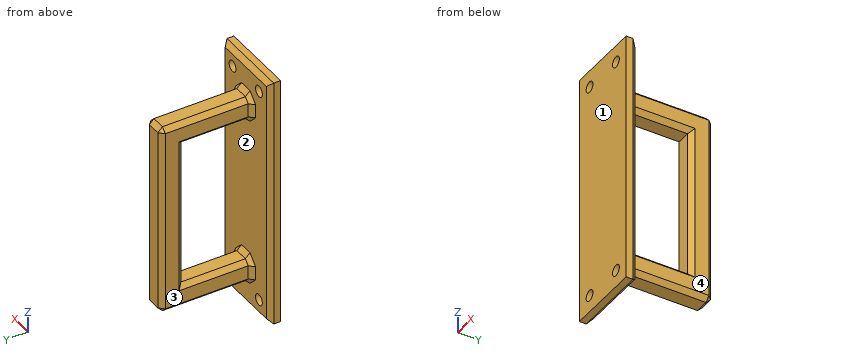
from build123d import *

# Parameters (mm, degrees)
SKETCH1_W           = 41.91
SKETCH1_H           = 139.7
BOSS_EXTRUDE1_DEPTH = 6.35
SKETCH2_R           = 3.048
CUT_EXTRUDE1_DEPTH  = 146.989248234
SKETCH3_W           = 12.7
SKETCH3_H           = 12.7
BOSS_EXTRUDE2_DEPTH = 50.8
BOSS_EXTRUDE3_REACH = 133.265
SKETCH4_W           = 12.7
SKETCH4_H           = 12.7
CHAMFER1_SIZE       = 2.54


with BuildPart() as part:
    # Sketch1 → Boss-Extrude1 (new body)
    with BuildSketch(Plane(origin=(0, 0, 0), x_dir=(1, 0, 0), z_dir=(0, 1, 0))):
        with Locations((-20.955, 69.85)):
            Rectangle(SKETCH1_W, SKETCH1_H)
    extrude(amount=BOSS_EXTRUDE1_DEPTH)

    # Sketch2 → Cut-Extrude1 (cut, through all)
    with BuildSketch(Plane(origin=(0, 6.35, 0), x_dir=(1, 0, 0), z_dir=(0, 1, 0))):
        with Locations(Location((-32.766, 130.302, 0), (0, 0, 270))):
            Circle(SKETCH2_R)
        with Locations(Location((-9.144, 130.302, 0), (0, 0, 270))):
            Circle(SKETCH2_R)
        with Locations(Location((-9.144, 9.398, 0), (0, 0, 270))):
            Circle(SKETCH2_R)
        with Locations(Location((-32.766, 9.398, 0), (0, 0, 270))):
            Circle(SKETCH2_R)
    extrude(amount=-CUT_EXTRUDE1_DEPTH, mode=Mode.SUBTRACT)

    # Sketch3 → Boss-Extrude2 (add)
    with BuildSketch(Plane(origin=(0, 6.35, 0), x_dir=(1, 0, 0), z_dir=(0, 1, 0))):
        with Locations((-20.955, 116.84)):
            Rectangle(SKETCH3_W, SKETCH3_H)
        with Locations((-20.955, 22.86)):
            Rectangle(SKETCH3_W, SKETCH3_H)
    extrude(amount=BOSS_EXTRUDE2_DEPTH)

    # Sketch4 → Boss-Extrude3 (add, up to next)
    with BuildSketch(Plane.XY.offset(-110.49), mode=Mode.PRIVATE) as boss_extrude3_sk1:
        with Locations((-20.955, 50.8)):
            Rectangle(SKETCH4_W, SKETCH4_H)
    boss_extrude3_tool1 = extrude(boss_extrude3_sk1.sketch, amount=BOSS_EXTRUDE3_REACH, mode=Mode.PRIVATE) - part.part
    add(boss_extrude3_tool1.solids().sort_by_distance((-20.955, 50.8, -110.49))[0])

    # Chamfer1
    chamfer1_edges = [part.edges().sort_by_distance(p)[0] for p in [
        (-41.91, 6.35, -69.85),
        (-20.955, 6.35, 0),
        (-27.305, 6.35, -116.84),
        (-27.305, 31.75, -123.19),
        (-20.955, 6.35, -110.49),
        (-14.605, 6.35, -116.84),
        (-20.955, 6.35, -123.19),
        (-14.605, 31.75, -123.19),
        (-27.305, 57.15, -69.85),
        (-14.605, 57.15, -69.85),
        (-20.955, 57.15, -123.19),
        (-27.305, 6.35, -22.86),
        (-20.955, 6.35, -16.51),
        (-27.305, 31.75, -16.51),
        (-14.605, 6.35, -22.86),
        (-14.605, 31.75, -16.51),
        (-20.955, 6.35, -29.21),
        (-20.955, 57.15, -16.51),
        (0, 6.35, -69.85),
        (-14.605, 25.4, -29.21),
        (-14.605, 25.4, -110.49),
        (-27.305, 25.4, -110.49),
        (-27.305, 25.4, -29.21),
        (-27.305, 44.45, -69.85),
        (-14.605, 44.45, -69.85),
        (-20.955, 6.35, -139.7),
    ]]
    chamfer(chamfer1_edges, length=CHAMFER1_SIZE)


solid = part.part
Geometry: final body of the model. Coordinates: model frame, mm. Face numbers are marked on the shaded views. A direction names the side the tool comes from. Coordinates: 2 decimals unless noted, no trailing zeros. Loops run counter-clockwise (first coordinate to the right, second up) from the corner with the lowest first, then second, coordinate; pieces in that order, holes last. Notation, with made-up numbers: (0, 84.5) - (6, 84.5) arc R3 ccw to (6, 89.5) - close; hole circle Ø10 at (-17, -6.75). An arc over 180 degrees is marked (long way). Put each result on its own line as item: value. Start each with the question number.
Q1. Pull-direction query (Z, two-part tool) for the marked faces 1 and 2; classes: released by +Z, released by -Z, zero draft, split by the parting line, or undercut.
Q2. Cut plane A-A, the plane y = 33.5. Return loops of the section in (x, z) (3 decimals).
Q3. Cut plane B-B, the plane z = -98.5. Return loops of the section in (x, y) (3 decimals), and give its area (3 significant figures).
Q4. Pin query (flat end, axial travel): pin 1 Ø4 at (x, y) = (-22, 35.5) entering from -Z; pin 2 Ø3 at (x, z) = (-30, -36.5) entering from +Y; pin 3 Ø3 at (x, y) = (-35.5, 7) entering from +Z; pin 4 Ø2.5 at (x, z) = (-19.5, -67) entering from -Y. Return the tip coordinate at first contact, or that it passes through.
Q5. Set-up query: the marked faces 3 and 4. Return all of +Z, -Z, +X, -X, +Y, -Y with unobstructed straight access to the full face (end or side cutting, diameter ignored); none if empty.
Q6. Cut plane C-C, the plane x = -21. Return loops of the section in (y, z).
Q7. Cut plane D-D, the plane z = -21.5. Return loops of the section in (x, y) (3 decimals), and give its area (3 significant figures).
Q8. Line query: line 1 (Z direction, x = -23, y = 33); line 2 (Y direction, x = -21, z = -48); line 3 (Y direction, x = -38, z = -114.5). Output: solid intervals per line, ascending.
Filled sheet:
1. face 1: zero draft
1. face 2: undercut
2. outline: (-27.305, -120.65) - (-24.765, -123.19) - (-17.145, -123.19) - (-14.605, -120.65) - (-14.605, -113.03) - (-17.145, -110.49) - (-24.765, -110.49) - (-27.305, -113.03) - close; (-27.305, -26.67) - (-24.765, -29.21) - (-17.145, -29.21) - (-14.605, -26.67) - (-14.605, -19.05) - (-17.145, -16.51) - (-24.765, -16.51) - (-27.305, -19.05) - close
3. outline: (-41.91, 0) - (0, 0) - (0, 3.81) - (-2.54, 6.35) - (-39.37, 6.35) - (-41.91, 3.81) - close; (-27.305, 46.99) - (-24.765, 44.45) - (-17.145, 44.45) - (-14.605, 46.99) - (-14.605, 54.61) - (-17.145, 57.15) - (-24.765, 57.15) - (-27.305, 54.61) - close
3. area: 408 mm²
4. pin 1: z = -123.19
4. pin 2: y = 6.35
4. pin 3: z = -1.69
4. pin 4: y = 0
5. face 3: +Z, -Z, -X, +Y
5. face 4: +Z, -Z, +X, +Y
6. outline: (0, -139.7) - (3.81, -139.7) - (6.35, -137.16) - (6.35, -125.73) - (8.89, -123.19) - (54.61, -123.19) - (57.15, -120.65) - (57.15, -19.05) - (54.61, -16.51) - (8.89, -16.51) - (6.35, -13.97) - (6.35, -2.54) - (3.81, 0) - (0, 0) - close; hole (6.35, -107.95) - (8.89, -110.49) - (44.45, -110.49) - (44.45, -29.21) - (8.89, -29.21) - (6.35, -31.75) - close
7. outline: (-41.91, 0) - (0, 0) - (0, 3.81) - (-2.54, 6.35) - (-12.065, 6.35) - (-14.605, 8.89) - (-14.605, 54.61) - (-17.145, 57.15) - (-24.765, 57.15) - (-27.305, 54.61) - (-27.305, 8.89) - (-29.845, 6.35) - (-39.37, 6.35) - (-41.91, 3.81) - close
7. area: 905 mm²
8. line 1: -123.19 to -110.49, -29.21 to -16.51
8. line 2: 0 to 6.35, 44.45 to 57.15
8. line 3: 0 to 6.35
